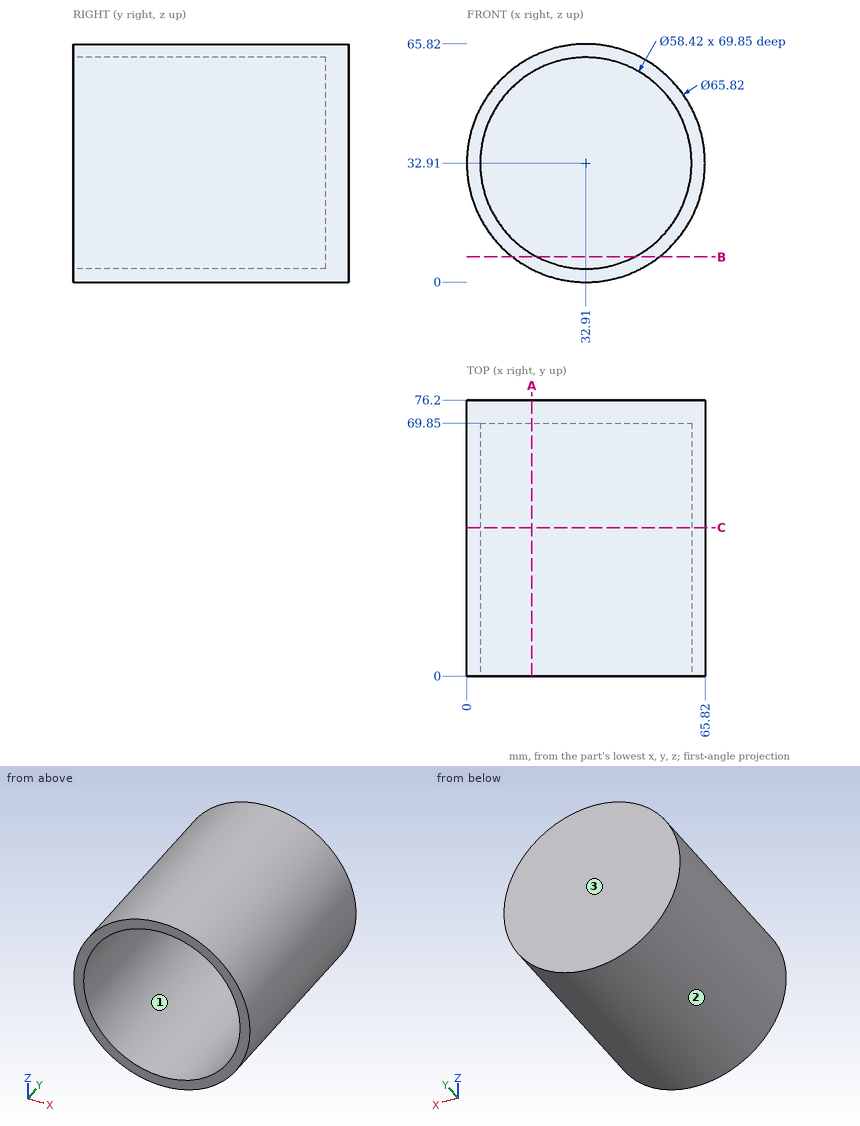
Here's the drawing with two shaded views (mm, measured from the low corner). I have some questions. Round coordinates to 2 decimals unless told otherwise and drop trailing zeros. Order: outer loops, then holes, each group sorted by start corner. A loop starts at its lowest first (then second) coordinate and runs counter-clockwise, first axis right, second up. Notation, with made-up numbers: (29.25, 49.5) -> (41.25, 49.5) arc R17 ccw to (41.25, 56.5) -> close; hole circle Ø10 at (37.5, -13.75). An arc over 180 degrees is marked (long way). Use a Markdown table: item, result. Add a question column.
(1) Suppose I cut it at A-A, the plane x = 18. Please give me the cut outline in (y, z).
(2) Suppose I cut it at C-C, the plane y = 41. Please give me the cut outline in (x, z), and give its area (3 significant figures).
(3) If we mould it in two halves opening along X, with no side actions, what happens to the marked faces 1, 2 and 3? For each: released by +X, released by -X, zero draft, split by the parting line, or undercut.
(4) Suppose I cut it at B-B, the plane z = 7. Please give me the cut outline in (x, y).
(5) I need wall thicknesses on line 1 along Z through (x, y) = (32, 43.5); line 2 along Y through (x, z) = (38, 28.5); line 3 along Z through (x, y) = (35, 25.5) (1 decimal). Which ranges of each line are inside material? Lowest first, please.
(6) For pin 1 Ø2 at (y, z) = (28, 44.5) entering from +X; pin 2 Ø5 at (x, y) = (48, 47.5) entering from +Z; pin 3 Ø5 at (y, z) = (49, 49.5) entering from -X, each with a flat end and sliding along its axis, tell me the tip position at first contact or that it passes through.
Verdict:
| question | item | result |
|---|---|---|
| 1 | outline | (0, 3.57) -> (76.2, 3.57) -> (76.2, 62.25) -> (0, 62.25) -> (0, 58.03) -> (69.85, 58.03) -> (69.85, 7.79) -> (0, 7.79) -> close |
| 2 | outline | circle Ø65.82 at (32.91, 32.91); hole circle Ø58.42 at (32.91, 32.91) |
| 2 | area | 722 mm2 |
| 3 | face 1 | undercut |
| 3 | face 2 | split by the parting line |
| 3 | face 3 | zero draft |
| 4 | outline | (12.62, 0) -> (19.42, 0) -> (19.42, 69.85) -> (46.4, 69.85) -> (46.4, 0) -> (53.2, 0) -> (53.2, 76.2) -> (12.62, 76.2) -> close |
| 5 | line 1 | 0.01 to 3.71, 62.11 to 65.81 |
| 5 | line 2 | 69.85 to 76.2 |
| 5 | line 3 | 0.1 to 3.8, 62 to 65.8 |
| 6 | pin 1 | x = 64.07 |
| 6 | pin 2 | z = 63.32 |
| 6 | pin 3 | x = 3.17 |
